from build123d import *

# Parameters (mm, degrees)
BOSS_EXTRUDE3_DEPTH      = 45
BOSS_EXTRUDE3_DEPTH_BACK = 45
SKETCH4_W                = 400
SKETCH4_H                = 200
BOSS_EXTRUDE9_DEPTH      = 50
BOSS_EXTRUDE9_DEPTH_BACK = 50
EXTRUDE_THIN1_START      = -380
EXTRUDE_THIN1_DEPTH      = 380
MIRROR6_START            = -380
MIRROR6_COPY_1_DEPTH     = 380
CUT_EXTRUDE5_DEPTH       = 243.950612345
MIRROR8_COPY_1_DEPTH     = 243.950612345
CUT_EXTRUDE6_DEPTH       = 1
CHAMFER2_SIZE            = 2
CHAMFER3_START           = -200
CHAMFER3_DEPTH           = 400
MIRROR11_COPY_1_DEPTH    = 1


with BuildPart() as part:
    # Sketch4 → Boss-Extrude3 (new, two sides: drawn at the far end of the back side and taken through both)
    with BuildSketch(Plane.XY.offset(-BOSS_EXTRUDE3_DEPTH_BACK)):
        Rectangle(SKETCH4_W, SKETCH4_H)
    extrude(amount=BOSS_EXTRUDE3_DEPTH + BOSS_EXTRUDE3_DEPTH_BACK)

    # Sketch5 → Boss-Extrude9 (add, two sides: drawn at the far end of the back side and taken through both)
    with BuildSketch(Plane.XY.offset(-BOSS_EXTRUDE9_DEPTH_BACK)):
        with BuildLine():
            ThreePointArc((2.236067977, -1.118033989), (0, -0.590169944), (-2.236067977, -1.118033989))
            Line((-2.236067977, -1.118033989), (-190, -95))
            Line((-190, -95), (-190, 95))
            Line((-190, 95), (-2.236067977, 1.118033989))
            ThreePointArc((-2.236067977, 1.118033989), (0, 0.590169944), (2.236067977, 1.118033989))
            Line((2.236067977, 1.118033989), (190, 95))
            Line((190, 95), (190, -95))
            Line((190, -95), (2.236067977, -1.118033989))
        make_face()
        with BuildLine():
            ThreePointArc((2.236067977, 1.118033989), (0, 0.590169944), (-2.236067977, 1.118033989))
            Line((-2.236067977, 1.118033989), (-190, 95))
            Line((-190, 95), (190, 95))
            Line((190, 95), (2.236067977, 1.118033989))
        make_face()
        with BuildLine():
            Line((2.236067977, -1.118033989), (190, -95))
            Line((190, -95), (-190, -95))
            Line((-190, -95), (-2.236067977, -1.118033989))
            ThreePointArc((-2.236067977, -1.118033989), (0, -0.590169944), (2.236067977, -1.118033989))
        make_face()
    extrude(amount=BOSS_EXTRUDE9_DEPTH + BOSS_EXTRUDE9_DEPTH_BACK)

    # Extrude-Thin1: read off the stored shape, not the designer's step
    # Extrude-Thin1 outline → Extrude-Thin1 (add)
    with BuildSketch(Plane.ZY.offset(190).offset(EXTRUDE_THIN1_START)):
        with BuildLine():
            add(Edge.make_bspline(
                [(-50, 95), (-48.146158838, 95), (-45.468843049, 95.640067172), (-45, 98.16553813), (-45, 100)],
                knots=[0, 0, 0, 0, 0.512954667, 1, 1, 1, 1], degree=3))
            Line((-50, 95), (-45, 95))
            Line((-45, 95), (-45, 100))
        make_face()
    extrude_thin1 = extrude(amount=EXTRUDE_THIN1_DEPTH)

    # Mirror5: Extrude-Thin1 across plane
    add(extrude_thin1.mirror(Plane.ZX))

    # Mirror6: Extrude-Thin1 across plane
    add(extrude_thin1.mirror(Plane.XY))

    # Mirror6 copy 1 sketch → Mirror6 copy 1 (add)
    with BuildSketch(Plane(origin=(-190, 0, 0), x_dir=(0, 0, -1), z_dir=(-1, 0, 0)).offset(MIRROR6_START)):
        with BuildLine():
            add(Edge.make_bspline(
                [(-50, 95), (-48.146158838, 95), (-45.468843049, 95.640067172), (-45, 98.16553813), (-45, 100)],
                knots=[0, 0, 0, 0, 0.512954667, 1, 1, 1, 1], degree=3))
            Line((-50, 95), (-45, 95))
            Line((-45, 95), (-45, 100))
        make_face()
    extrude(amount=MIRROR6_COPY_1_DEPTH)

    # Sketch11 → Cut-Extrude5 (cut, through all)
    with BuildSketch(Plane(origin=(0, 0, -45), x_dir=(-1, 0, 0), z_dir=(0, 0, -1))):
        Polygon((-197.710907072, 100), (-200, 97.710907072), (-200, 100), align=None)
    cut_extrude5 = extrude(amount=-CUT_EXTRUDE5_DEPTH, mode=Mode.SUBTRACT)

    # Mirror7: Cut-Extrude5 across plane
    add(cut_extrude5.mirror(Plane.ZX), mode=Mode.SUBTRACT)

    # Mirror8: Cut-Extrude5 across plane
    add(cut_extrude5.mirror(Plane(origin=(0, 0, 0), x_dir=(0, 0, 1), z_dir=(1, 0, 0))), mode=Mode.SUBTRACT)

    # Mirror8 copy 1 sketch → Mirror8 copy 1 (cut, through all)
    with BuildSketch(Plane(origin=(0, 0, -45), x_dir=(1, 0, 0), z_dir=(0, 0, -1))):
        Polygon((-197.710907072, 100), (-200, 97.710907072), (-200, 100), align=None)
    extrude(amount=-MIRROR8_COPY_1_DEPTH, mode=Mode.SUBTRACT)

    # Sketch12 → Cut-Extrude6 (cut)
    with BuildSketch(Plane(origin=(0, 0, -50), x_dir=(-1, 0, 0), z_dir=(0, 0, -1))):
        Polygon((-181.874897075, 89.170531546), (181.874897075, 89.170531546), (134.560480933, 32.233127844), (-112.917374812, 32.233127844), align=None)
    cut_extrude6 = extrude(amount=-CUT_EXTRUDE6_DEPTH, mode=Mode.SUBTRACT)

    # Mirror9: Cut-Extrude6 across plane
    add(cut_extrude6.mirror(Plane.ZX), mode=Mode.SUBTRACT)

    # Chamfer2
    chamfer2_edges = [part.edges().sort_by_distance(p)[0] for p in [
        (200, 0, 45),
        (200, 0, -45),
        (-200, 0, -45),
        (-200, 0, 45),
    ]]
    chamfer(chamfer2_edges, length=CHAMFER2_SIZE)

    # Chamfer3: read off the stored shape, not the designer's step
    # Chamfer3 outline → Chamfer3 (cut)
    with BuildSketch(Plane.YZ.offset(CHAMFER3_START)):
        with BuildLine():
            Line((-100, 45), (-100, 43))
            Line((-100, 43), (-97.823486796, 45.176513202))
            add(Edge.make_bspline(
                [(-97.823486796, 45.176513202), (-98.429622739, 45.049035026), (-99.14991283, 45), (-100, 45)],
                knots=[0.774303846, 0.774303846, 0.774303846, 0.774303846, 1, 1, 1, 1], degree=3))
        make_face()
        with BuildLine():
            Line((-100, -43), (-100, -45))
            add(Edge.make_bspline(
                [(-97.823486796, -45.176513202), (-98.429622739, -45.049035026), (-99.14991283, -45), (-100, -45)],
                knots=[0.774303846, 0.774303846, 0.774303846, 0.774303846, 1, 1, 1, 1], degree=3))
            Line((-97.823486796, -45.176513202), (-100, -43))
        make_face()
        with BuildLine():
            Line((100, 43), (100, 45))
            add(Edge.make_bspline(
                [(97.823486796, 45.176513202), (98.429622739, 45.049035026), (99.14991283, 45), (100, 45)],
                knots=[0.774303846, 0.774303846, 0.774303846, 0.774303846, 1, 1, 1, 1], degree=3))
            Line((97.823486796, 45.176513202), (100, 43))
        make_face()
        with BuildLine():
            add(Edge.make_bspline(
                [(97.823486796, -45.176513202), (98.429622739, -45.049035026), (99.14991283, -45), (100, -45)],
                knots=[0.774303846, 0.774303846, 0.774303846, 0.774303846, 1, 1, 1, 1], degree=3))
            Line((100, -45), (100, -43))
            Line((100, -43), (97.823486796, -45.176513202))
        make_face()
    extrude(amount=CHAMFER3_DEPTH, mode=Mode.SUBTRACT)

    # Mirror11: Cut-Extrude6 across plane
    add(cut_extrude6.mirror(Plane.XY), mode=Mode.SUBTRACT)

    # Mirror11 copy 1 sketch → Mirror11 copy 1 (cut)
    with BuildSketch(Plane(origin=(0, 0, 50), x_dir=(-1, 0, 0), z_dir=(0, 0, 1))):
        Polygon((-181.874897075, 89.170531546), (181.874897075, 89.170531546), (134.560480933, 32.233127844), (-112.917374812, 32.233127844), align=None)
    extrude(amount=-MIRROR11_COPY_1_DEPTH, mode=Mode.SUBTRACT)


solid = part.part
For this review, take the finished solid that the model builds, in its own axes (mm). A direction names the side the tool comes from. Round coordinates to 2 decimals unless told otherwise and drop trailing zeros. Order: outer loops, then holes, each group sorted by start corner. A loop starts at its lowest first (then second) coordinate and runs counter-clockwise, first axis right, second up. Notation, with made-up numbers: M -22,7 L -5,7 A26 cw -5,22 Z; hole C 55,-11 d10. An arc over 180 degrees is marked long. Write each question's results on one line, items separated by ' | '. Start each with the question number.
1. Draft analysis for pull direction Y (two halves, no side actions). For faces 1 (the face through (-3, 100, -1)), 2 (the face through (-158.55, -61.1, -49.51)), 3 (the face through (3, 1, -50)), state which applies: pulls with the +Y half, pulls with the -Y half, needs draft (parallel to the pull), parting line crosses it, or undercut.
2. Add section B-B (y = 74.5). State the section outline as (x, z) points, then the cut area to 3 significant figures.
3. Tool access review of faces 4 (the face through (-3, 61, 49)), 5 (the face through (-194, 1, -45)), 6 (the face through (-194, 1, 45)), 7 (the face through (194, 1, -45)): name each direction out of +Z, -Z, +X, -X, +Y, -Y from which nothing blocks a thin tool from reaching the whole face with its end or side.
4. Clearance check with flat-ended pins moving along their axes: pin 1 Ø0.5 at (x, z) = (-9, -49.5) entering from +Y; pin 2 Ø1.1 at (x, z) = (6, -49.5) entering from -Y; pin 3 Ø8 at (x, y) = (20.5, 54) entering from -Z. State where each tip first meets the part, or that it passes through.
5. Add section A-A (y = -79). State the section outline as (x, z) points.
6. To check wall thickness, follow L1, parallel to Z at x = -56.5, y = -36.5; L2, parallel to X at y = 10, z = 44. State the ranges of each line that lie inside material, in increasing order. Write a range as [from, to].
Output values:
1) face 1: pulls with the +Y half | face 2: undercut | face 3: needs draft
2) outline: M -200,-43 L -198,-45 L -190,-45 L -190,-50 L -169.68,-50 L -169.68,-49 L 164.11,-49 L 164.11,-50 L 190,-50 L 190,-45 L 198,-45 L 200,-43 L 200,43 L 198,45 L 190,45 L 190,50 L 164.11,50 L 164.11,49 L -169.68,49 L -169.68,50 L -190,50 L -190,45 L -198,45 L -200,43 Z | area: 39,100 mm^2
3) face 4: +Z | face 5: -Z, -X, +Y, -Y | face 6: +Z, -X, +Y, -Y | face 7: -Z, +X, +Y, -Y
4) pin 1: y = 95.02 | pin 2: y = -95.04 | pin 3: z = -49
5) outline: M -200,-43 L -198,-45 L -190,-45 L -190,-50 L -173.42,-50 L -173.42,-49 L 169.56,-49 L 169.56,-50 L 190,-50 L 190,-45 L 198,-45 L 200,-43 L 200,43 L 198,45 L 190,45 L 190,50 L 169.56,50 L 169.56,49 L -173.42,49 L -173.42,50 L -190,50 L -190,45 L -198,45 L -200,43 Z
6) L1: [-49, 49] | L2: [-199, 199]
